Could you check a few things on this model? Use its own coordinates, in mm. Round coordinates to 2 decimals unless told otherwise and drop trailing zeros. Write each loop counter-clockwise with the first axis right and the second up, starting at its lowest first coordinate (ties: lowest second). Pieces come first, ordered by that corner, then holes. Notation, with made-up numbers: (11, 70) -> (69, 70) arc R23 ccw to (69, 107) -> close; hole circle Ø6 at (70.5, 19). An arc over 180 degrees is marked (long way). Answer in a Markdown table with one row per item.
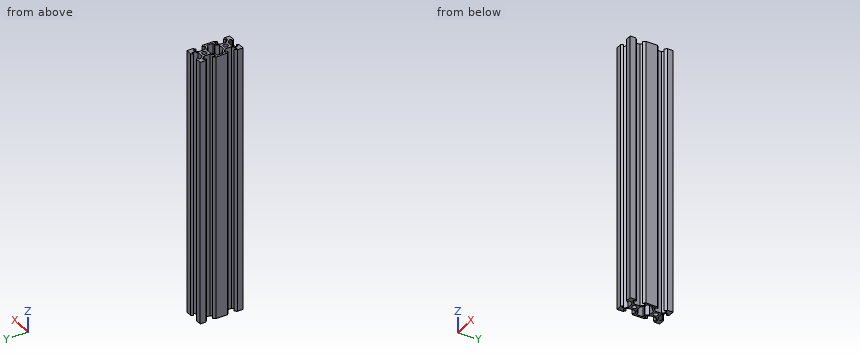
Autodesk Inventor part; units mm, degrees
ref_plane "YZ Plane" through (0, 0, 0) normal (1, 0, 0) x (0, 1, 0)
ref_plane "XZ Plane" through (0, 0, 0) normal (0, 1, 0) x (-1, 0, 0)
ref_plane "XY Plane" through (0, 0, 0) normal (0, 0, 1) x (1, 0, 0)
sketch "Sketch1" plane through (0, 0, 0) normal (0, 0, 1) x (1, 0, 0)
  line L0 (-3.9007, 3.9007) -> (3.9007, 3.9007)
  line L1 (3.9007, 3.9007) -> (3.9007, -3.9007)
  line L2 (3.9007, -3.9007) -> (-3.9007, -3.9007)
  line L3 (-3.9007, -3.9007) -> (-3.9007, 3.9007)
  line L4 (0, 3.9007) -> (0, -3.9007) construction
  line L5 (-3.9007, 0) -> (3.9007, 0) construction
  circle A0 centre (0, 0) radius 2.1
  line L6 (0, 0) -> (-16.1173, 16.1173) construction
  line L7 (0, 0) -> (22.7933, 0) construction
  line L8 (-2.84, 3.9007) -> (-5.4993, 6.56)
  line L9 (-5.4993, 6.56) -> (-5.4993, 8.2)
  line L10 (-5.4993, 8.2) -> (-2.84, 8.2)
  line L11 (-2.84, 8.2) -> (-4.64, 10)
  line L12 (-4.64, 10) -> (-10, 10)
  line L13 (-10, 10) -> (-10, 4.64)
  line L14 (-10, 4.64) -> (-8.2, 2.84)
  line L15 (-8.2, 2.84) -> (-8.2, 5.4993)
  line L16 (-8.2, 5.4993) -> (-6.56, 5.4993)
  line L17 (-6.56, 5.4993) -> (-3.9007, 2.84)
  line L18 (-3.9007, 2.84) -> (-11.3102, 2.84) construction
  line L19 (-2.84, 3.9007) -> (-3.9007, 3.9007)
  line L20 (-3.9007, 2.84) -> (-3.9007, 3.9007)
  line L21 (-3.9007, -2.84) -> (-6.56, -5.4993)
  line L22 (-6.56, -5.4993) -> (-8.2, -5.4993)
  line L23 (-8.2, -5.4993) -> (-8.2, -2.84)
  line L24 (-8.2, -2.84) -> (-10, -4.64)
  line L25 (-10, -4.64) -> (-10, -10)
  line L26 (-10, -10) -> (-4.64, -10)
  line L27 (-4.64, -10) -> (-2.84, -8.2)
  line L28 (-2.84, -8.2) -> (-5.4993, -8.2)
  line L29 (-5.4993, -8.2) -> (-5.4993, -6.56)
  line L30 (-5.4993, -6.56) -> (-2.84, -3.9007)
  line L31 (-3.9007, -2.84) -> (-3.9007, -3.9007)
  line L32 (-2.84, -3.9007) -> (-3.9007, -3.9007)
  line L33 (2.84, -3.9007) -> (5.4993, -6.56)
  line L34 (5.4993, -6.56) -> (5.4993, -8.2)
  line L35 (5.4993, -8.2) -> (2.84, -8.2)
  line L36 (2.84, -8.2) -> (4.64, -10)
  line L37 (4.64, -10) -> (10, -10)
  line L38 (10, -10) -> (10, -4.64)
  line L39 (10, -4.64) -> (8.2, -2.84)
  line L40 (8.2, -2.84) -> (8.2, -5.4993)
  line L41 (8.2, -5.4993) -> (6.56, -5.4993)
  line L42 (6.56, -5.4993) -> (3.9007, -2.84)
  line L43 (2.84, -3.9007) -> (3.9007, -3.9007)
  line L44 (3.9007, -2.84) -> (3.9007, -3.9007)
  line L45 (3.9007, 2.84) -> (6.56, 5.4993)
  line L46 (6.56, 5.4993) -> (8.2, 5.4993)
  line L47 (8.2, 5.4993) -> (8.2, 2.84)
  line L48 (8.2, 2.84) -> (10, 4.64)
  line L49 (10, 4.64) -> (10, 10)
  line L50 (10, 10) -> (4.64, 10)
  line L51 (4.64, 10) -> (2.84, 8.2)
  line L52 (2.84, 8.2) -> (5.4993, 8.2)
  line L53 (5.4993, 8.2) -> (5.4993, 6.56)
  line L54 (5.4993, 6.56) -> (2.84, 3.9007)
  line L55 (3.9007, 2.84) -> (3.9007, 3.9007)
  line L56 (2.84, 3.9007) -> (3.9007, 3.9007)
  dimension "d7" = 4.2
  dimension "d8" = 135
  dimension "d9" = 1.5
  dimension "d10" = 1.64
  dimension "d11" = 1.8
  dimension "d12" = 2.84
  dimension "d13" = 10
  dimension "d16" = 360
extrude "Extrusion1" add sketch "Sketch1" along normal blind 250
pattern_linear "Rectangular Pattern1" count 2 spacing 20 along (0, -1, 0) of "Extrusion1"
sketch "Sketch2" plane through (0, 0, 250) normal (0, 0, 1) x (1, 0, 0)
  line L0 (8.2, -2.84) -> (8.2, -5.4993)
  line L1 (8.2, -5.4993) -> (6.56, -5.4993)
  line L2 (-6.56, -5.4993) -> (-8.2, -5.4993)
  line L3 (-8.2, -5.4993) -> (-8.2, -2.84)
  line L4 (-8.2, -14.5007) -> (-6.56, -14.5007)
  line L5 (6.56, -14.5007) -> (8.2, -14.5007)
  line L6 (5.4993, -11.8) -> (5.4993, -13.44)
  line L7 (5.4993, -13.44) -> (2.84, -16.0993)
  line L8 (-2.84, -16.0993) -> (-5.4993, -13.44)
  line L9 (-5.4993, -8.2) -> (-5.4993, -6.56)
  line L10 (-5.4993, -6.56) -> (-2.84, -3.9007)
  line L11 (2.84, -3.9007) -> (5.4993, -6.56)
  line L12 (2.84, -8.2) -> (4.64, -10)
  line L13 (-8.2, -6.9993) -> (-5.9387, -6.9993)
  line L14 (-5.9387, -6.9993) -> (-4.1231, -5.1837)
  line L15 (-4.1231, -5.1837) -> (4.1231, -5.1837)
  line L16 (4.1231, -5.1837) -> (5.9387, -6.9993)
  line L17 (5.9387, -6.9993) -> (8.2, -6.9993)
  line L18 (8.2, -6.9993) -> (8.2, -13.0007)
  line L19 (8.2, -13.0007) -> (5.9387, -13.0007)
  line L20 (5.9387, -13.0007) -> (4.2461, -14.6932)
  line L21 (4.2461, -14.6932) -> (-4.2461, -14.6932)
  line L22 (-4.2461, -14.6932) -> (-5.9387, -13.0007)
  line L23 (-5.9387, -13.0007) -> (-8.2, -13.0007)
  line L24 (-8.2, -13.0007) -> (-8.2, -6.9993)
  dimension "d23" = 1.5
  dimension "d24" = 1.5
  dimension "d25" = 1.5
  dimension "d26" = 1.5
extrude "Extrusion2" cut sketch "Sketch2" against normal up to next
equation "\"d24\" = d23"
equation "\"d25\" = d23"
equation "\"d26\" = d23"
properties part number "20x40x250mm"
1) Please list where these lines run through material, in increasing order: line 1 (Y direction, x = 0, z = 198); line 2 (Y direction, x = -5.75, z = 64); line 3 (X direction, y = -4.5, z = 117.5).
Findings:
| item | result |
|---|---|
| line 1 | y = -23.9 to -22.1, -17.9 to -16.1, -3.9 to -2.1, 2.1 to 3.9 |
| line 2 | y = -30 to -24.69, -15.31 to -13.19, -6.81 to -4.69, 4.69 to 10 |
| line 3 | x = -9.86 to -8.2, -5.56 to -3.44, 3.44 to 5.56, 8.2 to 9.86 |
2) For pin 1 (3 mm diameter, centred on y = -19, z = 95, fed in from +X); pin 2 (1.7 mm diameter, centred on x = 1, z = 68, fed in from -Y); pin 3 (1.5 mm diameter, centred on y = -23.5, z = 120, fed in from +X), each with a flat end and sliding along its axis, tell me the tip position at first contact or that it passes through.
Findings:
| item | result |
|---|---|
| pin 1 | stops at x = 3.9 |
| pin 2 | stops at y = -23.9 |
| pin 3 | stops at x = 9.61 |
3) Imagine slicing it at A-A, the plane y = 0. Please give me the cut outline in (x, z).
Findings:
| item | result |
|---|---|
| outline | (-3.9, 0) -> (-2.1, 0) -> (-2.1, 250) -> (-3.9, 250) -> close; (2.1, 0) -> (3.9, 0) -> (3.9, 250) -> (2.1, 250) -> close |
4) Imagine slicing it at C-C, the plane z = 101. Count the separate pieces of the cut face and the enclosed holes in it, plus the area to 3 significant figures.
Findings:
| item | result |
|---|---|
| separate pieces | 1 |
| enclosed holes | 3 |
| area | 297 mm^2 |
5) Imagine slicing it at B-B, the plane x = 0. Please give me the cut outline in (y, z).
Findings:
| item | result |
|---|---|
| outline | (-23.9, 0) -> (-22.1, 0) -> (-22.1, 250) -> (-23.9, 250) -> close; (-17.9, 0) -> (-16.1, 0) -> (-16.1, 250) -> (-17.9, 250) -> close; (-3.9, 0) -> (-2.1, 0) -> (-2.1, 250) -> (-3.9, 250) -> close; (2.1, 0) -> (3.9, 0) -> (3.9, 250) -> (2.1, 250) -> close |
